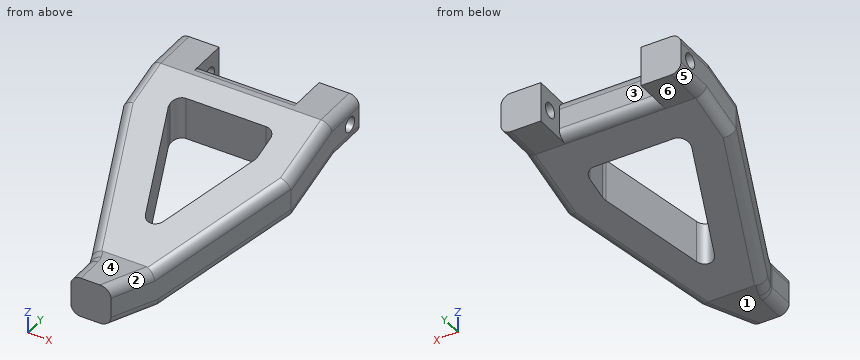
```python
from build123d import *

# Parameters (mm, degrees)
F1_DEPTH = 127
F3_DEPTH = 627.38
F5_DEPTH = 546.1
F6_R     = 19.05
F7_DEPTH = 409.956
F8_R     = 25.39999


# Not quite as in the source:
# - a fillet or chamfer is up to 0.001 mm smaller than in the source, because OpenCascade refuses the exact size


with BuildPart() as f1:
    # F0 (on Top) → F1 (new body, symmetric)
    with BuildSketch(Plane.XY):
        with BuildLine():
            Line((228.6, 73.2671543956), (228.6, 355.6))
            Line((228.6, 355.6), (127, 355.6))
            Line((127, 355.6), (127, 279.4))
            Line((127, 279.4), (-127, 279.4))
            Line((-127, 279.4), (-127, 355.6))
            Line((-127, 355.6), (-228.6, 355.6))
            Line((-228.6, 355.6), (-228.6, 127))
            Line((-228.6, 127), (-69.3541612572, -274.8921242948))
            ThreePointArc((-69.3541612572, -274.8921242948), (-68.0185057912, -279.4860093319), (-67.5679594278, -284.2488617581))
            Line((-67.5679594278, -284.2488617581), (-67.5679594278, -355.6))
            Line((-67.5679594278, -355.6), (34.0320405722, -355.6))
            Line((34.0320405722, -355.6), (228.6, 73.2671543956))
        make_face()
        with BuildLine():
            Line((126.9999997139, 152.3999997139), (126.9999997139, 100.7287641896))
            ThreePointArc((126.9999997139, 100.7287641896), (126.4262326875, 95.3605096932), (124.7308535455, 90.2347849149))
            Line((124.7308535455, 90.2347849149), (26.9491079367, -125.2959690409))
            ThreePointArc((26.9491079367, -125.2959690409), (3.2004851004, -140.194476085), (-19.7955440656, -124.1587272294))
            Line((-19.7955440656, -124.1587272294), (-125.2137978845, 141.8875713817))
            ThreePointArc((-125.2137978845, 141.8875713817), (-126.5494533505, 146.4814564188), (-126.9999997139, 151.244308845))
            Line((-126.9999997139, 151.244308845), (-126.9999997139, 152.3999997139))
            ThreePointArc((-126.9999997139, 152.3999997139), (-119.560511956, 170.360511956), (-101.5999997139, 177.7999997139))
            Line((-101.5999997139, 177.7999997139), (101.5999997139, 177.7999997139))
            ThreePointArc((101.5999997139, 177.7999997139), (119.560511956, 170.360511956), (126.9999997139, 152.3999997139))
        make_face(mode=Mode.SUBTRACT)
    extrude(amount=F1_DEPTH, both=True)

    # F2 (on face) → F3 (cut)
    with BuildSketch(Plane.YZ.offset(228.6)):
        Polygon((-228.6, -127), (-355.6, -127), (-355.6, -25.4), (-399.7474312782, -25.4), (-399.7474312782, -182.4822723866), (403.1273424625, -182.4822723866), (403.1273424625, 126.7705559731), (355.6, 127), (355.6, 25.4), (254, 25.4), align=None)
    extrude(amount=-F3_DEPTH, mode=Mode.SUBTRACT)

    # F4 (on face) → F5 (cut)
    with BuildSketch(Plane.YZ.offset(228.6)):
        Polygon((238.3390568884, 127), (355.6, 127), (355.6, 150.2672582865), (-388.3270025253, 150.2672582865), (-355.6, -25.4), (-244.2609431116, -25.4), (42.6722074132, 65.2104685868), align=None)
    extrude(amount=-F5_DEPTH, mode=Mode.SUBTRACT)

    # F6 (on face) → F7 (cut, symmetric)
    with BuildSketch(Plane.YZ.offset(-127)):
        with Locations((317.5, 76.2)):
            Circle(F6_R)
    extrude(amount=F7_DEPTH, both=True, mode=Mode.SUBTRACT)

    # F8 (radius 25.4 in the source; OpenCascade refuses exactly that, so slightly less here)
    f8_edges = [f1.edges().sort_by_distance(p)[0] for p in [
        (156.572108, -85.496894, 24.736015),
        (228.6, 155.803106, 100.936015),
        (228.6, 296.969528, 127),
        (59.288128, -299.930472, -25.4),
        (-67.567959, -319.924431, -25.4),
        (-155.045734, -58.630472, 33.220149),
        (-228.6, 182.669528, 109.420149),
        (-228.6, 296.969528, 127),
        (-228.6, 304.8, 25.4),
        (-228.6, 190.5, 5.347368),
        (-158.148482, -50.8, -70.852632),
        (-78.525563, -251.746062, -127),
        (-67.567959, -319.924431, -127),
        (160.124628, -77.666423, -79.336765),
        (62.840648, -292.1, -127),
        (228.6, 163.633577, -3.136765),
        (228.6, 304.8, 25.4),
        (0, 279.4, 127),
        (0, 279.4, 25.4),
    ]]
    fillet(f8_edges, radius=F8_R)


solid = f1.part
```
Input: part model. Units: mm. Frame: model coordinates. Face numbers are marked on the shaded views. A direction names the side the tool comes from. Give positions to 0.01 mm unless a question says otherwise; leave off trailing zeros. Write each loop counter-clockwise with the first axis right and the second up, starting at its lowest first coordinate (ties: lowest second). Pieces come first, ordered by that corner, then holes. Notation, with made-up numbers: (8, -21) - (28, -21) arc R18 ccw to (28, 10) - close; hole circle Ø3 at (73, -38.75). An arc over 180 degrees is marked (long way). Write item = value, one per line. Start each with the question number.
1) Cut plane A-A (y = 317.5). Return loops of the section in (x, z).
2) Pin query (flat end, axial travel): pin 1 (12 mm diameter, centred on x = 11.5, y = -143, fed in from +Z); pin 2 (6 mm diameter, centred on y = -182.5, z = -59.5, fed in from -X); pin 3 (5 mm diameter, centred on y = 110, z = -6, fed in from -X). Return the tip coordinate at first contact, or that it passes through.
3) Draft query along X for the marked faces 1, 2 and 3. Return one class per face: pulls with the +X half, pulls with the -X half, needs draft (parallel to the pull), parting line crosses it, or undercut.
4) Material intervals for L1, parallel to X at y = 327.5, z = 50.5; L2, parallel to Z at x = -190, y = 317; L3, parallel to Y at x = -73, z = 65.5, sorted ascending. Write a range as [from, to].
5) Reachability of the marked faces 4, 5 and 6 from +Z, -Z, +X, -X, +Y, -Y: full face, straight path, thin tool, end or side. Return the list, or none.
Answers follow:
q1.outline = (-228.6, 50.8) arc R25.4 ccw to (-203.2, 25.4) - (-127, 25.4) - (-127, 57.15) - (-228.6, 57.15) - close; (-228.6, 95.25) - (-127, 95.25) - (-127, 127) - (-203.2, 127) arc R25.4 ccw to (-228.6, 101.6) - close; (127, 25.4) - (203.2, 25.4) arc R25.4 ccw to (228.6, 50.8) - (228.6, 57.15) - (127, 57.15) - close; (127, 95.25) - (228.6, 95.25) - (228.6, 101.6) arc R25.4 ccw to (203.2, 127) - (127, 127) - close
q2.pin_1 = 8.21
q2.pin_2 = -107.15
q2.pin_3 = -218.65
q3.face_1 = needs draft
q3.face_2 = pulls with the +X half
q3.face_3 = undercut
q4.L1 = [-228.6, -127], [127, 228.6]
q4.L2 = [25.4, 57.16], [95.24, 127]
q4.L3 = [177.8, 279.4]
q5.face_4 = +Z, +X, -X, -Y
q5.face_5 = -Z, -X, +Y
q5.face_6 = -Z, +X, -X, +Y
